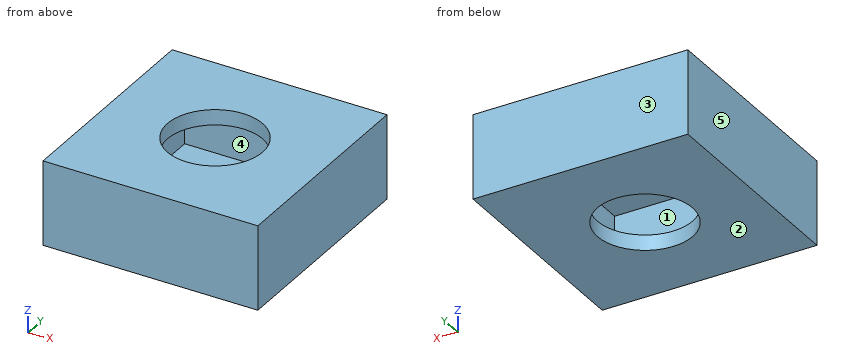
from build123d import *

# Parameters (mm, degrees)
F0_W     = 7
F0_H     = 7.1
F0_R     = 1.55
F1_DEPTH = 0.5
F2_W     = 7
F2_H     = 7.1
F2_W_2   = 5
F2_H_2   = 5.1
F3_DEPTH = 1.75
F4_W     = 7
F4_H     = 7.1
F4_R     = 1.55
F5_DEPTH = 0.5


with BuildPart() as f1:
    # F0 (on Top) → F1 (new body)
    with BuildSketch(Plane.XY):
        Rectangle(F0_W, F0_H)
        Circle(F0_R, mode=Mode.SUBTRACT)
    extrude(amount=F1_DEPTH)

    # F2 (on face) → F3 (join)
    with BuildSketch(Plane.XY.offset(0.5)):
        Rectangle(F2_W, F2_H)
        Rectangle(F2_W_2, F2_H_2, mode=Mode.SUBTRACT)
    extrude(amount=F3_DEPTH)

    # F4 (on face) → F5 (join)
    with BuildSketch(Plane.XY.offset(2.25)):
        Rectangle(F4_W, F4_H)
        Circle(F4_R, mode=Mode.SUBTRACT)
    extrude(amount=F5_DEPTH)


solid = f1.part
The listing builds one solid part. Answer for the finished solid, in the listing's coordinates (mm). Face numbers are marked on the shaded views. A direction names the side the tool comes from. Coordinates: 2 decimals unless noted, no trailing zeros. Write each loop counter-clockwise with the first axis right and the second up, starting at its lowest first coordinate (ties: lowest second). Pieces come first, ordered by that corner, then holes. Notation, with made-up numbers: (-35, -6) - (4, -6) arc R36 ccw to (4, 29) - close; hole circle Ø7 at (-35, -22.5). An arc over 180 degrees is marked (long way). Answer as CSV lines item,"result".
1. Find section D-D (z = 2). Give the vertices of the cut face in (x, y), plus the area to 3 significant figures.
Computed values:
outline,"(-3.5, -3.55) - (3.5, -3.55) - (3.5, 3.55) - (-3.5, 3.55) - close; hole (-2.5, -2.55) - (2.5, -2.55) - (2.5, 2.55) - (-2.5, 2.55) - close"
area,"24.2 mm²"
2. Given P1, Ø3, axis at x = 0, y = 0, coming from the +Z side, flat-ended and moving along its own axis, determine where the tip first touches the part or whether it passes through.
Computed values:
P1,"passes through"
3. Find section B-B (x = -2.25). Give the vertices of the cut face in (y, z), plus the area to 3 significant figures.
Computed values:
outline,"(-3.55, 0) - (3.55, 0) - (3.55, 2.75) - (-3.55, 2.75) - close; hole (-2.55, 0.5) - (2.55, 0.5) - (2.55, 2.25) - (-2.55, 2.25) - close"
area,"10.6 mm²"
4. Find section C-C (y = 0). Give the vertices of the cut face in (x, z), plus the area to 3 significant figures.
Computed values:
outline,"(-3.5, 0) - (-1.55, 0) - (-1.55, 0.5) - (-2.5, 0.5) - (-2.5, 2.25) - (-1.55, 2.25) - (-1.55, 2.75) - (-3.5, 2.75) - close; (1.55, 0) - (3.5, 0) - (3.5, 2.75) - (1.55, 2.75) - (1.55, 2.25) - (2.5, 2.25) - (2.5, 0.5) - (1.55, 0.5) - close"
area,"7.40 mm²"
5. Determine the mould class of the marked faces 3, 4 and 5 for opening direction X: +X half, -X half, draft (parallel to the pull), parting line (faces both ways), or undercut.
Computed values:
face 3,"draft"
face 4,"undercut"
face 5,"-X half"
6. Straight lines are drawn through the part: line 1 (Y direction, x = 0, z = 0.2); line 2 (Y direction, x = 2, z = 1.3); line 3 (Z direction, x = 1, y = -1.5). For each, find the intervals that lie inside material, in ascending order. Write a range as [from, to].
Computed values:
line 1,"y = [-3.55, -1.55], [1.55, 3.55]"
line 2,"y = [-3.55, -2.55], [2.55, 3.55]"
line 3,"z = [0, 0.5], [2.25, 2.75]"
7. A tool of negligible diameter and unlimited length cuts with its end or side. For the marked faces 1 and 2, from which of +Z, -Z, +X, -X, +Y, -Y can it reach the whole face along a straight path? Write none if from no direction.
Computed values:
face 1,"none"
face 2,"-Z, +X, -X, +Y, -Y"
8. Find section A-A (x = 0). Give the vertices of the cut face in (y, z).
Computed values:
outline,"(-3.55, 0) - (-1.55, 0) - (-1.55, 0.5) - (-2.55, 0.5) - (-2.55, 2.25) - (-1.55, 2.25) - (-1.55, 2.75) - (-3.55, 2.75) - close; (1.55, 0) - (3.55, 0) - (3.55, 2.75) - (1.55, 2.75) - (1.55, 2.25) - (2.55, 2.25) - (2.55, 0.5) - (1.55, 0.5) - close"
